The listing builds one solid part. Answer for the finished solid, in the listing's coordinates (mm). Face numbers are marked on the shaded views. A direction names the side the tool comes from. Coordinates: 2 decimals unless noted, no trailing zeros. Loops run counter-clockwise (first coordinate to the right, second up) from the corner with the lowest first, then second, coordinate; pieces in that order, holes last. Notation, with made-up numbers: (-8, -25) -> (36, -25) arc R15 ccw to (36, -17) -> close; hole circle Ø10 at (-7, 73). An arc over 180 degrees is marked (long way). Answer in a Markdown table with one row per item.
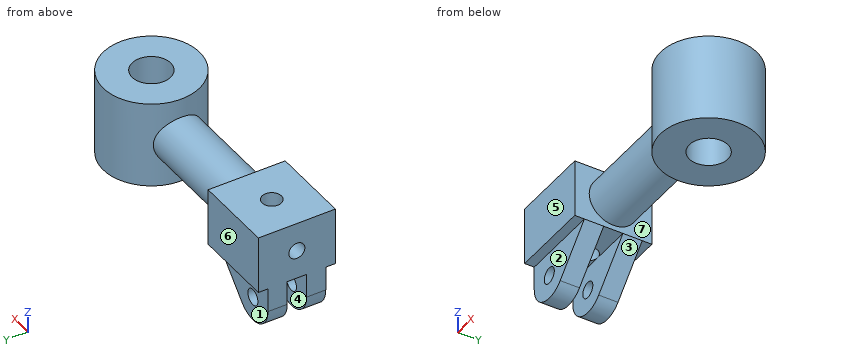
```python
from build123d import *

# Parameters (mm, degrees)
F0_R      = 30
F0_R_2    = 12
F1_DEPTH  = 54
F2_W      = 50
F2_H      = 36
F3_DEPTH  = 24
F6_W      = 120
F6_H      = 15
F8_R      = 6
F9_DEPTH  = 36
F10_R     = 5
F11_DEPTH = 21.6843753096
F13_R     = 5
F14_DEPTH = 12
F16_R     = 12
F17_DEPTH = 75.001


with BuildPart() as f1:
    # F0 (on Top) → F1 (new body)
    with BuildSketch(Plane.XY):
        Circle(F0_R)
        Circle(F0_R_2, mode=Mode.SUBTRACT)
    extrude(amount=F1_DEPTH)



with BuildPart() as f3:
    # F2 (on Front) → F3 (new body, symmetric)
    with BuildSketch(Plane.XZ):
        with Locations((-120, 27)):
            Rectangle(F2_W, F2_H)
    extrude(amount=F3_DEPTH, both=True)


with BuildPart() as f1_1:
    add(f1.part)

    add(f3.part)  # F7 merges F3
    # F6 (on offset) → F7 (revolve)
    with BuildSketch(Plane.XY.offset(27)):
        with Locations((-60, -7.5)):
            Rectangle(F6_W, F6_H)
    revolve(axis=Axis((-60, 0, 27), (1, 0, 0)))

    # F8 (on face) → F9 (cut, through all)
    with BuildSketch(Plane.XY.offset(45)):
        with Locations((-120, 0)):
            Circle(F8_R)
    extrude(amount=-F9_DEPTH, mode=Mode.SUBTRACT)

    # F10 (on face) → F11 (cut, through all)
    with BuildSketch(Plane(origin=(-145, 0, 0), x_dir=(0, -1, 0), z_dir=(-1, 0, 0))):
        with Locations((0, 27)):
            Circle(F10_R)
    extrude(amount=-F11_DEPTH, mode=Mode.SUBTRACT)

    # F13 (on offset) → F14 (join)
    with BuildSketch(Plane.XZ.offset(18)):
        with BuildLine():
            Line((-119.1379310345, -16.3448275862), (-95, 9))
            Line((-95, 9), (-145, 9))
            Line((-145, 9), (-145, -6))
            ThreePointArc((-145, -6), (-135.5708601453, -19.9271503633), (-119.1379310345, -16.3448275862))
        make_face()
        with Locations((-130, -6)):
            Circle(F13_R, mode=Mode.SUBTRACT)
    extrude(amount=-F14_DEPTH)

    # F15: F1 across plane


with BuildPart() as f1_2:
    add(f1_1.part)
    add(f1_1.part.mirror(Plane.XZ))

    # F16 (on face) → F17 (cut, through all)
    with BuildSketch(Plane.XY.offset(54)):
        Circle(F16_R)
    extrude(amount=-F17_DEPTH, mode=Mode.SUBTRACT)


solid = f1_2.part
```
Item 1: A cutting plane is placed at A-A, the plane x = -130. Determine the outline of the cut face in (y, z), plus the area to 3 significant figures.
Findings below:
| item | result |
|---|---|
| outline | (-24, 9) -> (-18, 9) -> (-18, -1) -> (-6, -1) -> (-6, 9) -> (6, 9) -> (6, -1) -> (18, -1) -> (18, 9) -> (24, 9) -> (24, 45) -> (-24, 45) -> close; (-18, -21) -> (-6, -21) -> (-6, -11) -> (-18, -11) -> close; (6, -21) -> (18, -21) -> (18, -11) -> (6, -11) -> close; hole circle Ø10 at (0, 27) |
| area | 2,130 mm2 |
Item 2: Determine the mould class of the marked faces 4, 5, 6 and 7 for opening direction Y: +Y half, -Y half, draft (parallel to the pull), parting line (faces both ways), or undercut.
Findings below:
| item | result |
|---|---|
| face 4 | undercut |
| face 5 | -Y half |
| face 6 | +Y half |
| face 7 | draft |
Item 3: Find the intervals of material crossed by probe 1 along Y at (x, z) = (-135, 7.5); probe 2 along X at (y, z) = (0.5, 43); probe 3 along Y at (x, z) = (-120, 29), in increasing order.
Findings below:
| item | result |
|---|---|
| probe 1 | y = -18 to -6, 6 to 18 |
| probe 2 | x = -145 to -125.98, -114.02 to -95, -30 to -11.99, 11.99 to 30 |
| probe 3 | y = -24 to -6, 6 to 24 |
Item 4: A cutting plane is placed at C-C, the plane y = 10. Determine the outline of the cut face in (x, z).
Findings below:
| item | result |
|---|---|
| outline | (-145, -6) arc R15 ccw to (-119.14, -16.34) -> (-95, 9) -> (-95, 15.82) -> (-28.28, 15.82) -> (-28.28, 0) -> (-6.63, 0) -> (-6.63, 54) -> (-28.28, 54) -> (-28.28, 38.18) -> (-95, 38.18) -> (-95, 45) -> (-145, 45) -> close; (6.63, 0) -> (28.28, 0) -> (28.28, 54) -> (6.63, 54) -> close; hole circle Ø10 at (-130, -6) |
Item 5: Flat-ended cylindrical pins translate along their axes: pin 1 Ø10 at (x, z) = (9.5, 17.5) entering from -Y; pin 2 Ø3 at (x, y) = (-115, -22) entering from -Z; pin 3 Ø9 at (x, z) = (-130, -1) entering from -Y; pin 4 Ø6 at (y, z) = (-13.5, 46) entering from -X. Find the tip coordinate at first contact, or state that the pin passes through.
Findings below:
| item | result |
|---|---|
| pin 1 | stops at y = -29.66 |
| pin 2 | stops at z = 9 |
| pin 3 | stops at y = -18 |
| pin 4 | stops at x = -145 |
Item 6: A cutting plane is placed at B-B, the plane z = 27. Determine the outline of the cut face in (x, y), plus the area to 3 significant figures.
Findings below:
| item | result |
|---|---|
| outline | (-145, -24) -> (-95, -24) -> (-95, -15) -> (-25.98, -15) arc R30 ccw (long way) to (-25.98, 15) -> (-95, 15) -> (-95, 24) -> (-145, 24) -> (-145, 5) -> (-123.32, 5) arc R6 cw (long way) to (-123.32, -5) -> (-145, -5) -> close; hole circle Ø24 at (0, 0) |
| area | 6,450 mm2 |
Item 7: A tool of negligible diameter and unlimited length cuts with its end or side. For the marked faces 1, 2 and 3, from which of +Z, -Z, +X, -X, +Y, -Y can it reach the whole face along a straight path? Write none if from no direction.
Findings below:
| item | result |
|---|---|
| face 1 | -Z, -X, +Y |
| face 2 | -Z, -X, -Y |
| face 3 | -Z, +Y, -Y |
Item 8: A cutting plane is placed at D-D, the plane y = -20. Determine the outline of the cut face in (x, z), plus the area to 3 significant figures.
Findings below:
| item | result |
|---|---|
| outline | (-145, 9) -> (-95, 9) -> (-95, 45) -> (-145, 45) -> close; (-22.36, 0) -> (22.36, 0) -> (22.36, 54) -> (-22.36, 54) -> close |
| area | 4,210 mm2 |
